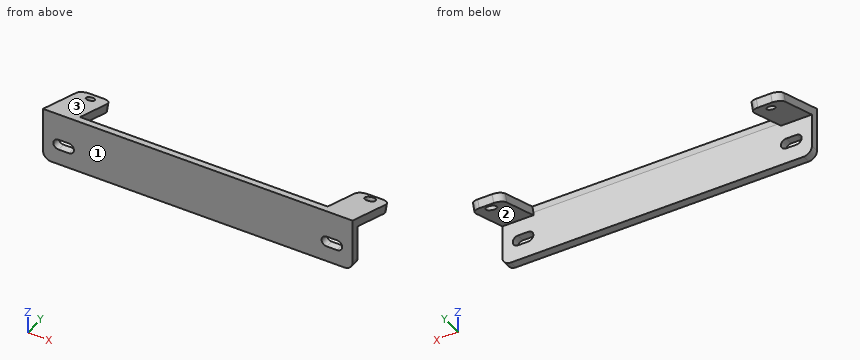
from build123d import *

# Parameters (mm, degrees)
SKETCH1_W           = 150
SKETCH1_H           = 20
BOSS_EXTRUDE1_DEPTH = 4
BOSS_EXTRUDE3_DEPTH = 150
SKETCH4_R           = 2.005
SKETCH4_R_2         = 2.5
SKETCH4_W           = 120
SKETCH4_H           = 26.389234781
CUT_EXTRUDE1_DEPTH  = 10
FILLET1_R           = 4
BOSS_EXTRUDE4_DEPTH = 150
CUT_EXTRUDE4_DEPTH  = 10


with BuildPart() as part:
    # Sketch1 → Boss-Extrude1 (new body)
    with BuildSketch(Plane(origin=(0, 0, 0), x_dir=(1, 0, 0), z_dir=(0, 1, 0))):
        Rectangle(SKETCH1_W, SKETCH1_H)
        with BuildLine():
            Line((-67.5, 2.5), (-62.5, 2.5))
            ThreePointArc((-62.5, 2.5), (-60, 0), (-62.5, -2.5))
            Line((-62.5, -2.5), (-67.5, -2.5))
            ThreePointArc((-67.5, -2.5), (-70, 0), (-67.5, 2.5))
        make_face(mode=Mode.SUBTRACT)
        with BuildLine():
            Line((62.5, 2.5), (67.5, 2.5))
            ThreePointArc((67.5, 2.5), (70, 0), (67.5, -2.5))
            Line((67.5, -2.5), (62.5, -2.5))
            ThreePointArc((62.5, -2.5), (60, 0), (62.5, 2.5))
        make_face(mode=Mode.SUBTRACT)
    extrude(amount=BOSS_EXTRUDE1_DEPTH)

    # Sketch3 → Boss-Extrude3 (add)
    with BuildSketch(Plane(origin=(75, 0, 0), x_dir=(0, 0, -1), z_dir=(1, 0, 0))):
        Polygon((-10, 0), (-15.416556228, 0), (-6.181619296, 30), (-2.358652574, 28.823171448), (-10, 4), align=None)
    extrude(amount=-BOSS_EXTRUDE3_DEPTH)

    # Sketch4 → Cut-Extrude1 (cut)
    with BuildSketch(Plane(origin=(0, 4.334920159, 14.082132419), x_dir=(1, 0, 0), z_dir=(0, 0.2942071381037286, 0.9557416805229401))):
        with Locations(Location((-67.5, 21.853573894, 0), (0, 0, 270))):
            Circle(SKETCH4_R)
        with Locations(Location((67.5, 22.843573894, 0), (0, 0, 270))):
            Circle(SKETCH4_R_2)
        with Locations((0, 13.658956504)):
            Rectangle(SKETCH4_W, SKETCH4_H)
    extrude(amount=-CUT_EXTRUDE1_DEPTH, mode=Mode.SUBTRACT)

    # Fillet1
    fillet1_edges = [part.edges().sort_by_distance(p)[0] for p in [
        (75, 29.411585724, 4.270135935),
        (-75, 29.411585724, 4.270135935),
        (-60, 29.411585724, 4.270135935),
        (60, 29.411585724, 4.270135935),
        (-75, 2, -10),
        (75, 2, -10),
    ]]
    fillet(fillet1_edges, radius=FILLET1_R)

    # Sketch5 → Boss-Extrude4 (add)
    with BuildSketch(Plane(origin=(75, 0, 0), x_dir=(0, 0, -1), z_dir=(1, 0, 0))):
        Polygon((6, 4), (6, 0), (-15.416556228, 0), (-14.185231304, 4), align=None)
    extrude(amount=-BOSS_EXTRUDE4_DEPTH)

    # Sketch7 → Cut-Extrude4 (cut)
    with BuildSketch(Plane.XZ):
        with BuildLine():
            Line((-62.5, -2.5), (-67.5, -2.5))
            ThreePointArc((-67.5, -2.5), (-70, 0), (-67.5, 2.5))
            Line((-67.5, 2.5), (-62.5, 2.5))
            ThreePointArc((-62.5, 2.5), (-60, 0), (-62.5, -2.5))
        make_face()
        with BuildLine():
            Line((62.5, 2.5), (67.5, 2.5))
            ThreePointArc((67.5, 2.5), (70, 0), (67.5, -2.5))
            Line((67.5, -2.5), (62.5, -2.5))
            ThreePointArc((62.5, -2.5), (60, 0), (62.5, 2.5))
        make_face()
    extrude(amount=-CUT_EXTRUDE4_DEPTH, mode=Mode.SUBTRACT)


solid = part.part
Here's how the part is built. I have some questions about the finished solid (model axes, mm). Face numbers are marked on the shaded views. Give positions to 0.01 mm unless a question says otherwise; leave off trailing zeros. Loops run counter-clockwise (first coordinate to the right, second up) from the corner with the lowest first, then second, coordinate; pieces in that order, holes last. Notation, with made-up numbers: (-33, -27) -> (-6, -27) arc R29 cw to (-6, -7) -> close; hole circle Ø1 at (-35.75, -22). An arc over 180 degrees is marked (long way). Answer as a JSON object with one key per item and string values. Group by question number.
Item 1: Thinking about a two-plate mould opening in Y: for the marked faces 1, 2 and 3, which applies, pulls with the +Y half, pulls with the -Y half, needs draft (parallel to the pull), parting line crosses it, or undercut?
Item 2: Imagine slicing it at B-B on y = 10. Write out the boundary of the cut face in (x, z), then the cut area to 3 significant figures.
Item 3: Will these pins go through, and if not, where does the flat tip stop? pin 1 (8 mm diameter, centred on x = -4.5, z = 8, fed in from -Y); pin 2 (1.2 mm diameter, centred on x = -65, y = 2.5, fed in from +Z); pin 3 (10 mm diameter, centred on x = 15.5, z = -6, fed in from +Y); pin 4 (3 mm diameter, centred on x = 64, y = 2, fed in from +Z).
Item 4: I need wall thicknesses on L1, parallel to X at y = 12, z = 11.25; L2, parallel to Y at x = 12, z = -5; L3, parallel to X at y = 24, z = 7.75. Which ranges of each line are inside material? Lowest first, please.
Item 5: Imagine slicing it at C-C on x = 29.5. Write out the boundary of the cut face in (y, z), then the cut area to 3 significant figures.
Item 6: Imagine slicing it at D-D on z = -7.75. Write out the boundary of the cut face in (x, y).
Item 7: Imagine slicing it at A-A on z = 0. Write out the boundary of the cut face in (x, y), then the cut area to 3 significant figures.
Answer list:
{
 "1": {"face 1": "pulls with the -Y half", "face 2": "undercut", "face 3": "pulls with the +Y half"},
 "2": {"outline": "(-75, 8.15) -> (-60, 8.15) -> (-60, 12.34) -> (-75, 12.34) -> close; (60, 8.15) -> (75, 8.15) -> (75, 12.34) -> (60, 12.34) -> close", "area": "126 mm2"},
 "3": {"pin 1": "stops at y = 0", "pin 2": "stops at z = 14.83", "pin 3": "stops at y = 4", "pin 4": "stops at z = 15.26"},
 "4": {"L1": "x = -75 to -60, 60 to 75", "L2": "y = 0 to 4", "L3": "x = -75 to -69.11, -65.89 to -60, 60 to 66.29, 68.71 to 75"},
 "5": {"outline": "(0, -10) -> (4, -10) -> (4, 11.42) -> (4.78, 13.95) -> (0, 15.42) -> close", "area": "100 mm2"},
 "6": {"outline": "(-74.6, 0) -> (74.6, 0) -> (74.6, 4) -> (-74.6, 4) -> close"},
 "7": {"outline": "(-75, 0) -> (-70, 0) -> (-70, 4) -> (-75, 4) -> close; (-60, 0) -> (60, 0) -> (60, 4) -> (-60, 4) -> close; (70, 0) -> (75, 0) -> (75, 4) -> (70, 4) -> close", "area": "520 mm2"}
}
